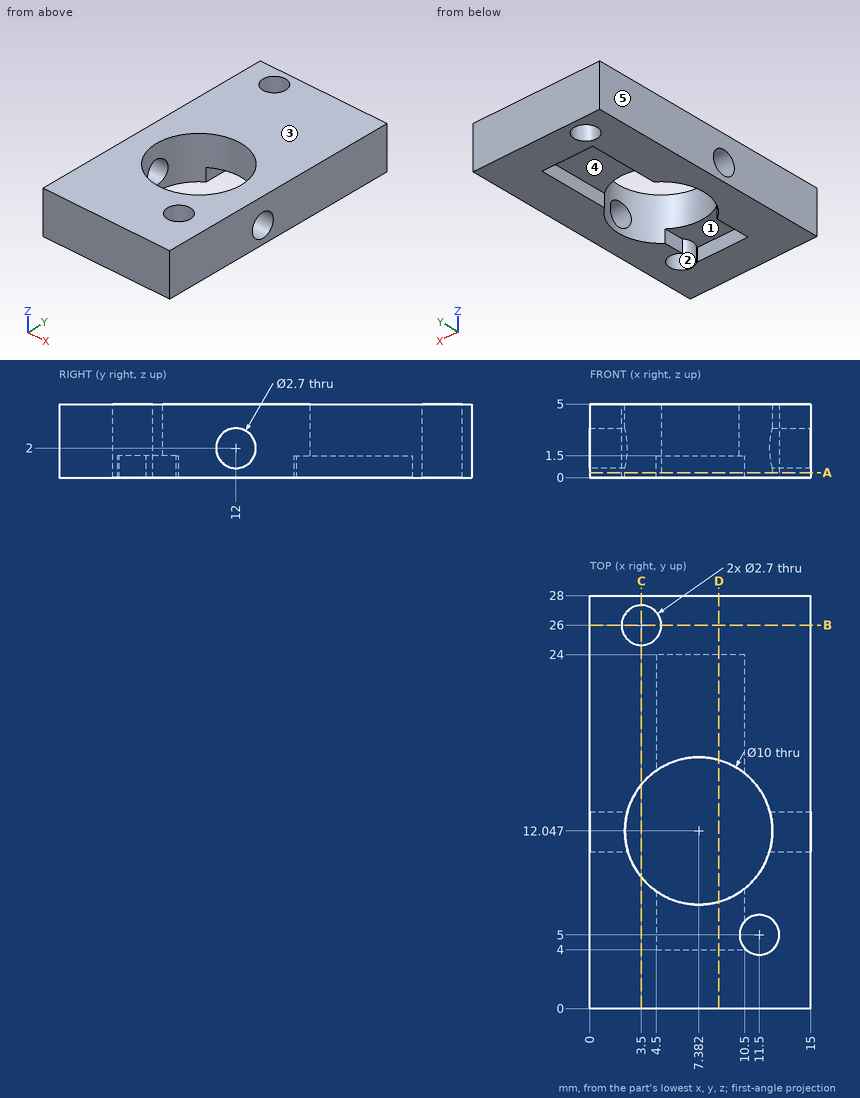
Design review of the part shown in the three views and the two pictorial views. Dimensions are in mm from the part's minimum x, y and z. A direction names the side the tool comes from. Give positions to 0.01 mm unless a question says otherwise; leave off trailing zeros. Loops run counter-clockwise (first coordinate to the right, second up) from the corner with the lowest first, then second, coordinate; pieces in that order, holes last. Notation, with made-up numbers: M 41.5,11.5 L 98.5,11.5 A12 ccw 98.5,30.5 Z; hole C 7.25,-15.5 d6. An arc over 180 degrees is marked long. Answer as a JSON object with one key per item and string values. Group by question number.
Q1. Mouldability with a two-part tool opening along X and no side actions: class the marked faces 3, 4 and 5 as +X half, -X half, draft (parallel to the pull), parting line (faces both ways), or undercut.
Q2. Add section B-B on y = 26. Give the boundary of the cut face in (x, z), and give its area (3 significant figures).
Q3. Add section D-D on x = 8.75. Give the boundary of the cut face in (y, z).
Q4. For probe 1 along X at (y, z) = (23.75, 1); probe 2 along Y at (x, z) = (13.95, 2); probe 3 along Y at (x, z) = (8.5, 1.25), list the stretches that pass through material, from the lowest coordinate up. Write a range as [from, to].
Q5. Add section C-C on x = 3.5. Give the boundary of the cut face in (y, z), and give its area (3 significant figures).
Q6. Tool access review of the marked faces 1 and 2: name each direction out of +Z, -Z, +X, -X, +Y, -Y from which nothing blocks a thin tool from reaching the whole face with its end or side.
Q7. Insertion check: P1, Ø9, axis at x = 7.38, y = 12.05, coming from the -Z side; P2, Ø2, axis at x = 7.5, y = 5.5, coming from the -Z side. Each pin has a flat end and moves straight along its axis. Give the tip position at first contact, or say it passes through.
Q8. Add section A-A on z = 0.35. Give the boundary of the cut face in (x, y).
Checked values:
{
 "1": {"face 3": "draft", "face 4": "undercut", "face 5": "-X half"},
 "2": {"outline": "M 0,0 L 2.15,0 L 2.15,5 L 0,5 Z; M 4.85,0 L 15,0 L 15,5 L 4.85,5 Z", "area": "61.5 mm²"},
 "3": {"outline": "M 0,0 L 4,0 L 4,1.5 L 7.24,1.5 L 7.24,5 L 0,5 Z; M 16.86,1.5 L 24,1.5 L 24,0 L 28,0 L 28,5 L 16.86,5 Z"},
 "4": {"probe 1": "[0, 4.5], [10.5, 15]", "probe 2": "[0, 10.65], [13.35, 28]", "probe 3": "[0, 4], [24, 28]"},
 "5": {"outline": "M 0,0 L 8.9,0 L 8.9,5 L 0,5 Z; M 15.2,0 L 24.65,0 L 24.65,5 L 15.2,5 Z; M 27.35,0 L 28,0 L 28,5 L 27.35,5 Z", "area": "95.0 mm²"},
 "6": {"face 1": "-Z", "face 2": "+Z, -Z"},
 "7": {"P1": "through", "P2": "z = 1.5"},
 "8": {"outline": "M 0,0 L 15,0 L 15,28 L 0,28 Z; hole C 3.5,26 d2.7; hole M 4.5,4 L 10.5,4 L 10.5,4.09 A1.35 ccw long 10.5,5.91 L 10.5,8.14 A5 ccw 10.5,15.96 L 10.5,24 L 4.5,24 L 4.5,16.13 A5 ccw 4.5,7.96 Z"}
}
